from build123d import *

# Parameters (mm, degrees)
SKETCH_W        = 100
SKETCH_H        = 25
PAD_DEPTH       = 21.5
SKETCH001_R     = 18.7
POCKET_DEPTH    = 25.001
SKETCH002_R     = 21.2
POCKET001_DEPTH = 3
SKETCH003_R     = 2
POCKET002_DEPTH = 21.501
POCKET003_DEPTH = 6


with BuildPart() as part:
    # Sketch → Pad (new body)
    with BuildSketch(Plane.XY):
        Rectangle(SKETCH_W, SKETCH_H)
    extrude(amount=PAD_DEPTH)

    # Sketch001 → Pocket (cut, through all)
    with BuildSketch(Plane.XZ.offset(12.5)):
        with Locations((0, 24.25)):
            Circle(SKETCH001_R)
    extrude(amount=-POCKET_DEPTH, mode=Mode.SUBTRACT)

    # Sketch002 → Pocket001 (cut)
    with BuildSketch(Plane.XZ.offset(12.5)):
        with Locations((0, 24.25)):
            Circle(SKETCH002_R)
    extrude(amount=-POCKET001_DEPTH, mode=Mode.SUBTRACT)

    # Sketch003 → Pocket002 (cut, through all)
    with BuildSketch(Plane(origin=(0, 0, 0), x_dir=(1, 0, 0), z_dir=(0, 0, -1))):
        with Locations((-35, -2.5)):
            Circle(SKETCH003_R)
        with Locations((35, -2.5)):
            Circle(SKETCH003_R)
    extrude(amount=-POCKET002_DEPTH, mode=Mode.SUBTRACT)

    # Sketch004 → Pocket003 (cut)
    with BuildSketch(Plane(origin=(0, 0, 0), x_dir=(1, 0, 0), z_dir=(0, 0, -1))):
        Polygon((-4.231557, 5.724423), (-4.877122, 7.393728), (-6.645565, 7.669305), (-7.768443, 6.275577), (-7.122878, 4.606272), (-5.354435, 4.330695), align=None)
        Polygon((6.393216, 4.253943), (7.708738, 5.467507), (7.315521, 7.213564), (5.606784, 7.746057), (4.291262, 6.532493), (4.684479, 4.786436), align=None)
        Polygon((-5.632013, -7.751548), (-4.299122, -6.557088), (-4.667109, -4.80554), (-6.367987, -4.248452), (-7.700878, -5.442912), (-7.332891, -7.19446), align=None)
        Polygon((6.905144, -7.544036), (7.789747, -5.98814), (6.884602, -4.444104), (5.094856, -4.455964), (4.210253, -6.01186), (5.115398, -7.555896), align=None)
    extrude(amount=-POCKET003_DEPTH, mode=Mode.SUBTRACT)


solid = part.part
The model under review builds one solid part; all positions refer to its coordinate system, in mm. A direction names the side the tool comes from. Round coordinates to 2 decimals unless told otherwise and drop trailing zeros. Loops run counter-clockwise (first coordinate to the right, second up) from the corner with the lowest first, then second, coordinate; pieces in that order, holes last. Notation, with made-up numbers: (29.25, -12) -> (69.25, -12) arc R23 cw to (69.25, 2) -> close; hole circle Ø8 at (68.5, 24). An arc over 180 degrees is marked (long way). Write item = value, one per line. Start each with the question number.
Item 1: Take a section at C-C on x = 35. Give the boundary of the cut face in (y, z), plus the area to 4 significant figures.
Item 2: Insertion check: pin 1 (1.7 mm diameter, centred on x = -6, y = -5.5, fed in from -Z); pin 2 (5.5 mm diameter, centred on x = -1, z = 10.5, fed in from -Y). Each pin has a flat end and moves straight along its axis. Give the tip position at first contact, or say it passes through.
Item 3: Take a section at A-A on y = 2.5. Give the boundary of the cut face in (x, z), plus the area to 3 significant figures.
Item 4: Take a section at D-D on y = -2. Give the boundary of the cut face in (x, z).
Item 5: Take a section at B-B on z = 13. Give the boundary of the cut face in (x, y), plus the area to 3 significant figures.
Item 6: Mouldability with a two-part tool opening along X and no side actions: class faces 1 (the flat face through (-1, 12.5, 3)), 2 (the flat face through (-50, 0, 11)), 3 (the flat face through (-6, -6, 6)) as released by +X, released by -X, zero draft, split by the parting line, or undercut.
Item 7: For faces 4 (the flat face through (-4.48, 5.69, 2.96)), 5 (the cylindrical face through (-0.428, -11.021, 3.054)), 6 (the cylindrical face through (-33.153, 3.266, 10.599)), list the 3-axis set-ups (+Z, -Z, +X, -X, +Y, -Y) from which the entire face can be reached by the end or side of a thin tool; tool diameter is ignored.
Item 8: To check wall thickness, follow L1, parallel to X at y = 2.5, z = 4.75; L2, parallel to Y at x = 35, z = 4.5; L3, parallel to X at y = 2.5, z = 7.5. State the ranges of each line that lie inside material, in increasing order.
Result:
q1.outline = (-12.5, 0) -> (0.5, 0) -> (0.5, 21.5) -> (-12.5, 21.5) -> close; (4.5, 0) -> (12.5, 0) -> (12.5, 21.5) -> (4.5, 21.5) -> close
q1.area = 451.5 mm²
q2.pin_1 = 6
q2.pin_2 = through
q3.outline = (-50, 0) -> (-37, 0) -> (-37, 21.5) -> (-50, 21.5) -> close; (-33, 0) -> (33, 0) -> (33, 21.5) -> (18.5, 21.5) arc R18.7 cw to (-18.5, 21.5) -> (-33, 21.5) -> close; (37, 0) -> (50, 0) -> (50, 21.5) -> (37, 21.5) -> close
q3.area = 1,530 mm²
q4.outline = (-50, 0) -> (50, 0) -> (50, 21.5) -> (18.5, 21.5) arc R18.7 cw to (-18.5, 21.5) -> (-50, 21.5) -> close
q5.outline = (-50, -12.5) -> (-17.97, -12.5) -> (-17.97, -9.5) -> (-14.94, -9.5) -> (-14.94, 12.5) -> (-50, 12.5) -> close; (14.94, -9.5) -> (17.97, -9.5) -> (17.97, -12.5) -> (50, -12.5) -> (50, 12.5) -> (14.94, 12.5) -> close; hole circle Ø4 at (-35, 2.5); hole circle Ø4 at (35, 2.5)
q5.area = 1,710 mm²
q6.face_1 = zero draft
q6.face_2 = released by -X
q6.face_3 = undercut
q7.face_4 = -Z
q7.face_5 = +Z, -Y
q7.face_6 = +Z, -Z
q8.L1 = -50 to -37, -33 to 33, 37 to 50
q8.L2 = -12.5 to 0.5, 4.5 to 12.5
q8.L3 = -50 to -37, -33 to -8.31, 8.31 to 33, 37 to 50
